Job drawing, mm, ordinate dimensions from the low corner. One solid piece. Coordinates: 2 decimals unless noted, no trailing zeros. Loops run counter-clockwise (first coordinate to the right, second up) from the corner with the lowest first, then second, coordinate; pieces in that order, holes last. Notation, with made-up numbers: (68.25, 73) - (101.25, 73) arc R18 cw to (101.25, 84) - close; hole circle Ø9 at (56, -29). An arc over 180 degrees is marked (long way). Use a Markdown table: item, result. Add a question column.
1. Wall check: probe 1 along Y at (x, z) = (56.9, 9.5); probe 2 along X at (y, z) = (114.5, 9.5); probe 3 along Y at (x, z) = (20.5, 11). Give the ranges that are in metal, low to high. Write a range as [from, to].
2. Band-saw the part on D-D, the plane x = 34.5. Give the cut face in (y, z), plus the area to 3 significant figures.
3. Band-saw the part on C-C, the plane z = 6.5. Give the cut face in (x, y).
4. Drop a flat-ended pin along its axis: pin 1 (1.5 mm diameter, centred on x = 23.5, z = 10.5, fed in from -Y). Give the stop position or say it passes through.
5. Band-saw the part on B-B, the plane y = 33.2. Give the cut face in (x, z).
6. Pull direction Y, two halves, no side cores. Call the marked faces 1, 2, 3 and 4: pulls with the +Y half, pulls with the -Y half, needs draft (parallel to the pull), parting line crosses it, or undercut.
7. Band-saw the part on A-A, the plane y = 9.5. Give the cut face in (x, z), plus the area to 3 significant figures.
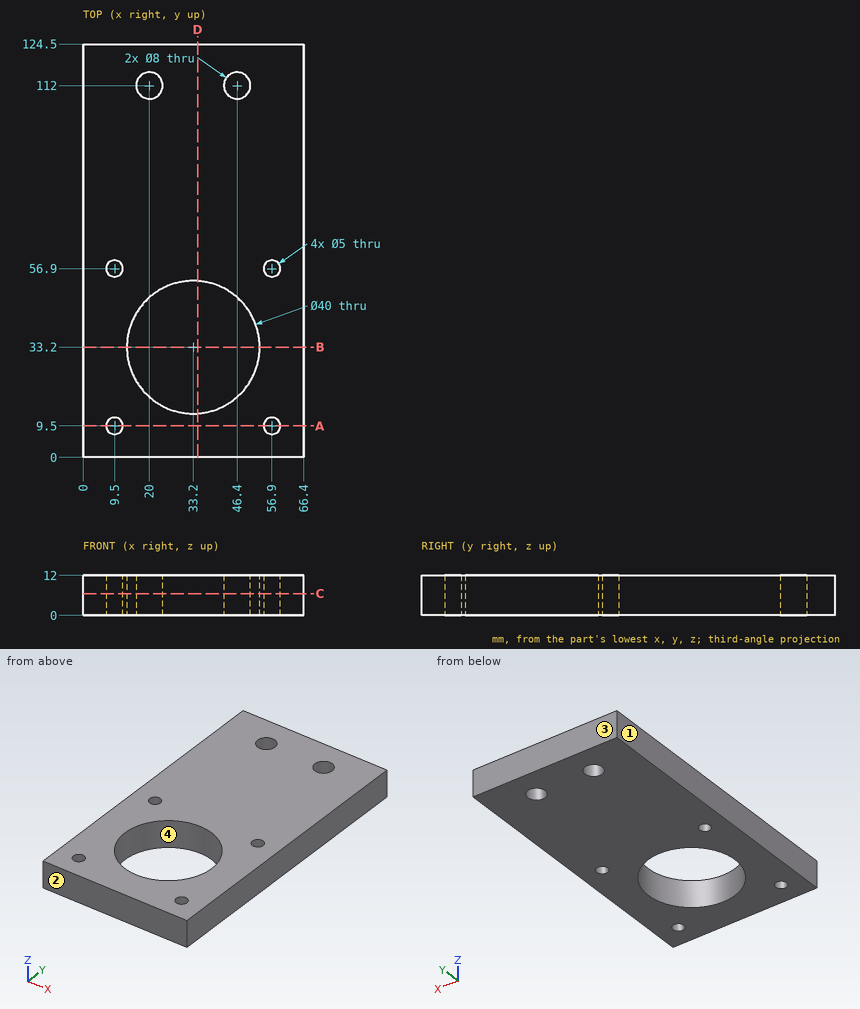
Geometry check:
| question | item | result |
|---|---|---|
| 1 | probe 1 | y = [0, 7], [12, 54.4], [59.4, 124.5] |
| 1 | probe 2 | x = [0, 16.88], [23.12, 43.28], [49.52, 66.4] |
| 1 | probe 3 | y = [0, 17.75], [48.65, 108.03], [115.97, 124.5] |
| 2 | outline | (0, 0) - (13.24, 0) - (13.24, 12) - (0, 12) - close; (53.16, 0) - (124.5, 0) - (124.5, 12) - (53.16, 12) - close |
| 2 | area | 1,020 mm^2 |
| 3 | outline | (0, 0) - (66.4, 0) - (66.4, 124.5) - (0, 124.5) - close; hole circle Ø5 at (9.5, 9.5); hole circle Ø5 at (9.5, 56.9); hole circle Ø40 at (33.2, 33.2); hole circle Ø8 at (20, 112); hole circle Ø8 at (46.4, 112); hole circle Ø5 at (56.9, 9.5); hole circle Ø5 at (56.9, 56.9) |
| 4 | pin 1 | stops at y = 0 |
| 5 | outline | (0, 0) - (13.2, 0) - (13.2, 12) - (0, 12) - close; (53.2, 0) - (66.4, 0) - (66.4, 12) - (53.2, 12) - close |
| 6 | face 1 | needs draft |
| 6 | face 2 | pulls with the -Y half |
| 6 | face 3 | pulls with the +Y half |
| 6 | face 4 | undercut |
| 7 | outline | (0, 0) - (7, 0) - (7, 12) - (0, 12) - close; (12, 0) - (54.4, 0) - (54.4, 12) - (12, 12) - close; (59.4, 0) - (66.4, 0) - (66.4, 12) - (59.4, 12) - close |
| 7 | area | 677 mm^2 |
